Part print with two shaded views. Sizes in mm from the minimum x, y, z corner. A direction names the side the tool comes from. Round coordinates to 2 decimals unless told otherwise and drop trailing zeros. Loops run counter-clockwise (first coordinate to the right, second up) from the corner with the lowest first, then second, coordinate; pieces in that order, holes last. Notation, with made-up numbers: (71, 75.25) - (122, 75.25) arc R27 ccw to (122, 92.25) - close; hole circle Ø7 at (4, -19.75). An arc over 180 degrees is marked (long way). Use a Markdown table: item, result.
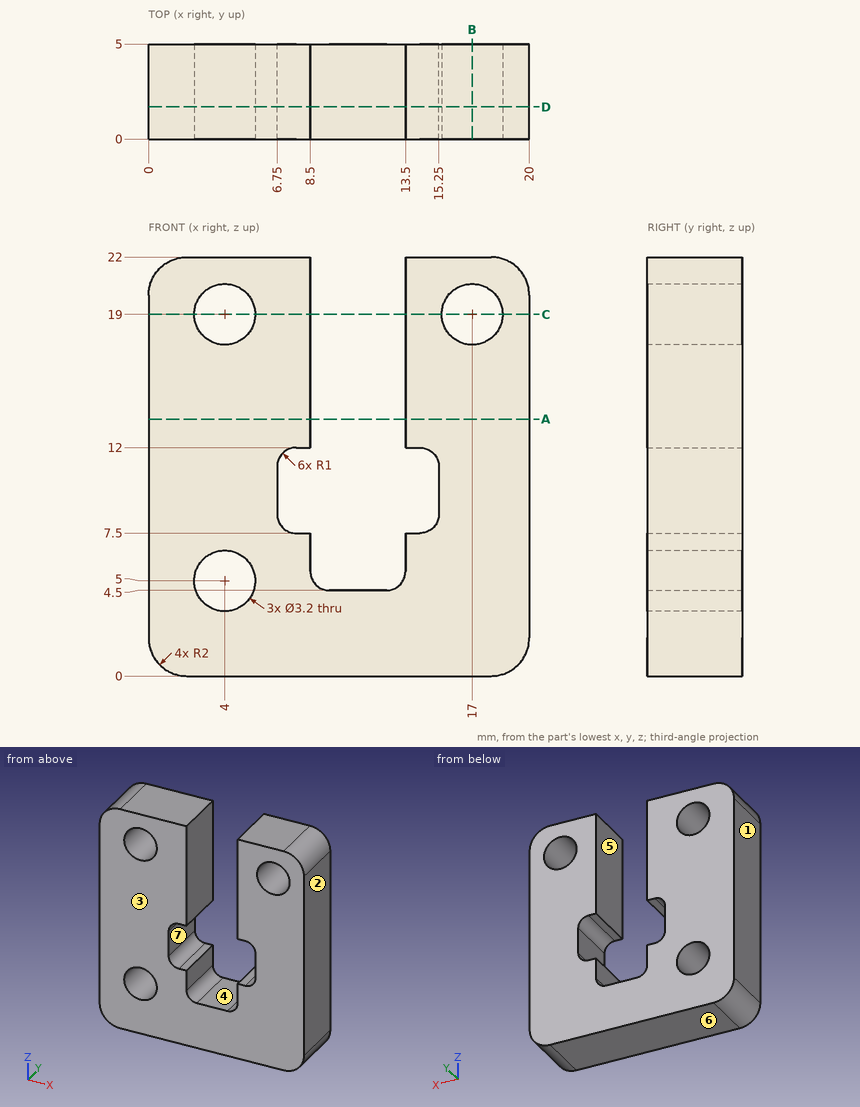
Q1. Probe line 1 (X direction, y = 2.1, z = 19); line 2 (X direction, y = 4.65, z = 12.5); line 3 (X direction, y = 1.35, z = 10). List the from-to ranges inside material, lowest first.
Results found:
| item | result |
|---|---|
| line 1 | x = 0 to 2.4, 5.6 to 8.5, 13.5 to 15.4, 18.6 to 20 |
| line 2 | x = 0 to 8.5, 13.5 to 20 |
| line 3 | x = 0 to 6.75, 15.25 to 20 |
Q2. Which spindle directions (+Z, -Z, +X, -X, +Y, -Y) get a long thin tool onto all of the face, cutting with end or side? Do the marked faces 5, 6 and 7. Say none if no direction does.
Results found:
| item | result |
|---|---|
| face 5 | +Z, +Y, -Y |
| face 6 | -Z, +X, -X, +Y, -Y |
| face 7 | +Y, -Y |
Q3. Drop flat-ended pins along their axis: pin 1 (2.5 mm diameter, centred on x = 11, y = 2.5, fed in from +Z); pin 2 (1.9 mm diameter, centred on x = 4, z = 5, fed in from -Y). Give the stop position or say it passes through.
Results found:
| item | result |
|---|---|
| pin 1 | stops at z = 4.5 |
| pin 2 | passes through |
Q4. Cut at C-C, the plane z = 19. List the corners of the cut face in (x, y), plus the area to 3 significant figures.
Results found:
| item | result |
|---|---|
| outline | (0, 0) - (2.4, 0) - (2.4, 5) - (0, 5) - close; (5.6, 0) - (8.5, 0) - (8.5, 5) - (5.6, 5) - close; (13.5, 0) - (15.4, 0) - (15.4, 5) - (13.5, 5) - close; (18.6, 0) - (20, 0) - (20, 5) - (18.6, 5) - close |
| area | 43.0 mm2 |
Q5. Pull direction X, two halves, no side cores. Call the marked faces 1, 2, 3 and 4: pulls with the +X half, pulls with the -X half, needs draft (parallel to the pull), parting line crosses it, or undercut.
Results found:
| item | result |
|---|---|
| face 1 | pulls with the -X half |
| face 2 | pulls with the +X half |
| face 3 | needs draft |
| face 4 | undercut |
Q6. Cut at B-B, the plane x = 17. List the corners of the cut face in (y, z), plus the area to 3 significant figures.
Results found:
| item | result |
|---|---|
| outline | (0, 0) - (5, 0) - (5, 17.4) - (0, 17.4) - close; (0, 20.6) - (5, 20.6) - (5, 22) - (0, 22) - close |
| area | 94.0 mm2 |
Q7. Cut at D-D, the plane y = 1.7. Count the separate pieces of the cut face and the enclosed holes in it, plus the area to 3 significant figures.
Results found:
| item | result |
|---|---|
| separate pieces | 1 |
| enclosed holes | 3 |
| area | 310 mm2 |
Q8. Cut at A-A, the plane z = 13.5. List the corners of the cut face in (x, y).
Results found:
| item | result |
|---|---|
| outline | (0, 0) - (8.5, 0) - (8.5, 5) - (0, 5) - close; (13.5, 0) - (20, 0) - (20, 5) - (13.5, 5) - close |
